CAD build for the part. Positions are in the model's coordinates, mm. A direction names the side the tool comes from. Round coordinates to 2 decimals unless told otherwise and drop trailing zeros. Write each loop counter-clockwise with the first axis right and the second up, starting at its lowest first coordinate (ties: lowest second). Pieces come first, ordered by that corner, then holes. Notation, with made-up numbers: (16, 12.5) - (53, 12.5) arc R19 ccw to (53, 22.5) - close; hole circle Ø1 at (46, 56.5). An arc over 180 degrees is marked (long way). Answer in a Markdown table with one row per item.
```python
from build123d import *

# Parameters (mm, degrees)
SKETCH1_W           = 42.291
SKETCH1_H           = 33.02
BOSS_EXTRUDE1_DEPTH = 42.418
FILLET1_R           = 2.54
SKETCH2_R           = 2.5273
BOSS_EXTRUDE2_DEPTH = 23.9649
CUT_EXTRUDE2_DEPTH  = 18.288
CUT_EXTRUDE3_REACH  = 58.985


with BuildPart() as part:
    # Sketch1 → Boss-Extrude1 (new body)
    with BuildSketch(Plane.XY):
        Rectangle(SKETCH1_W, SKETCH1_H)
    extrude(amount=BOSS_EXTRUDE1_DEPTH)

    # Fillet1
    fillet1_edges = [part.edges().sort_by_distance(p)[0] for p in [
        (21.1455, 0, 42.418),
        (0, 16.51, 42.418),
        (-21.1455, 0, 42.418),
        (0, 16.51, 0),
        (21.1455, 0, 0),
        (0, -16.51, 0),
        (-21.1455, 0, 0),
        (0, -16.51, 42.418),
        (-21.1455, 16.51, 21.209),
        (21.1455, 16.51, 21.209),
        (21.1455, -16.51, 21.209),
        (-21.1455, -16.51, 21.209),
    ]]
    fillet(fillet1_edges, radius=FILLET1_R)

    # Sketch2 → Boss-Extrude2 (add)
    with BuildSketch(Plane(origin=(0, 16.51, 0), x_dir=(1, 0, 0), z_dir=(0, 1, 0))):
        with Locations((0, -21.209)):
            Circle(SKETCH2_R)
    extrude(amount=BOSS_EXTRUDE2_DEPTH)

    # Sketch4 → Cut-Extrude2 (cut)
    with BuildSketch(Plane(origin=(0, 40.4749, 0), x_dir=(1, 0, 0), z_dir=(0, 1, 0))):
        with BuildLine():
            Line((-1.778, -23.005096125), (-1.778, -19.412903875))
            ThreePointArc((-1.778, -19.412903875), (-2.5273, -21.209), (-1.778, -23.005096125))
        make_face()
    extrude(amount=-CUT_EXTRUDE2_DEPTH, mode=Mode.SUBTRACT)

    # Sketch5 → Cut-Extrude3 (cut, up to next)
    with BuildSketch(Plane.XZ.offset(16.51), mode=Mode.PRIVATE) as cut_extrude3_sk1:
        Polygon((-21.1455, 42.418), (-21.1455, 38.107477062), (-16.834977062, 42.418), align=None)
    cut_extrude3_tool1 = extrude(cut_extrude3_sk1.sketch, amount=-CUT_EXTRUDE3_REACH, mode=Mode.PRIVATE) & part.part
    add(cut_extrude3_tool1.solids().sort_by_distance((-19.708659, -16.51, 40.981159))[0], mode=Mode.SUBTRACT)
    # Sketch5 → Cut-Extrude3 (cut, up to next)
    with BuildSketch(Plane.XZ.offset(16.51), mode=Mode.PRIVATE) as cut_extrude3_sk2:
        Polygon((16.961977062, 42.418), (21.2725, 38.107477062), (21.2725, 42.418), align=None)
    cut_extrude3_tool2 = extrude(cut_extrude3_sk2.sketch, amount=-CUT_EXTRUDE3_REACH, mode=Mode.PRIVATE) & part.part
    add(cut_extrude3_tool2.solids().sort_by_distance((19.835659, -16.51, 40.981159))[0], mode=Mode.SUBTRACT)
    # Sketch5 → Cut-Extrude3 (cut, up to next)
    with BuildSketch(Plane.XZ.offset(16.51), mode=Mode.PRIVATE) as cut_extrude3_sk3:
        Polygon((-21.1455, 0), (-16.834977062, 0), (-21.1455, 4.310522938), align=None)
    cut_extrude3_tool3 = extrude(cut_extrude3_sk3.sketch, amount=-CUT_EXTRUDE3_REACH, mode=Mode.PRIVATE) & part.part
    add(cut_extrude3_tool3.solids().sort_by_distance((-19.708659, -16.51, 1.436841))[0], mode=Mode.SUBTRACT)
    # Sketch5 → Cut-Extrude3 (cut, up to next)
    with BuildSketch(Plane.XZ.offset(16.51), mode=Mode.PRIVATE) as cut_extrude3_sk4:
        Polygon((21.2725, 0), (21.2725, 4.310522938), (16.961977062, 0), align=None)
    cut_extrude3_tool4 = extrude(cut_extrude3_sk4.sketch, amount=-CUT_EXTRUDE3_REACH, mode=Mode.PRIVATE) & part.part
    add(cut_extrude3_tool4.solids().sort_by_distance((19.835659, -16.51, 1.436841))[0], mode=Mode.SUBTRACT)


solid = part.part
```
Q1. Saw through at C-C on x = 0. List the corners of the cut face in (y, z).
Computed:
| item | result |
|---|---|
| outline | (-16.51, 2.54) arc R2.54 ccw to (-13.97, 0) - (13.97, 0) arc R2.54 ccw to (16.51, 2.54) - (16.51, 18.68) - (40.47, 18.68) - (40.47, 23.74) - (16.51, 23.74) - (16.51, 39.88) arc R2.54 ccw to (13.97, 42.42) - (-13.97, 42.42) arc R2.54 ccw to (-16.51, 39.88) - close |
Q2. Saw through at B-B on y = -10.5. List the corners of the cut face in (x, z), then the cut area to 3 significant figures.
Computed:
| item | result |
|---|---|
| outline | (-21.15, 4.31) - (-16.83, 0) - (16.96, 0) - (21.15, 4.18) - (21.15, 38.23) - (16.96, 42.42) - (-16.83, 42.42) - (-21.15, 38.11) - close |
| area | 1,760 mm2 |
Q3. Drill centre lines: line 1 (Y direction, x = 15, z = 40.5); line 2 (Y direction, x = 4.5, z = 29.5); line 3 (X direction, y = 4.5, z = 39). Where is each one in solid material? Low to high.
Computed:
| item | result |
|---|---|
| line 1 | y = -16.43 to 16.43 |
| line 2 | y = -16.51 to 16.51 |
| line 3 | x = -20.25 to 20.38 |
Q4. Flat gauge pins, fed straight in: pin 1 (10 mm diameter, centred on x = -16, y = 20.5, fed in from -Z); pin 2 (1.1 mm diameter, centred on y = 31.5, z = 21, fed in from -X); pin 3 (10 mm diameter, centred on x = -15.5, z = 16.5, fed in from +Y); pin 4 (0.6 mm diameter, centred on x = -2, z = 20.5, fed in from +Y). Where does each tip first touch, or does it go through?
Computed:
| item | result |
|---|---|
| pin 1 | stops at z = 0.51 |
| pin 2 | stops at x = -1.78 |
| pin 3 | stops at y = 16.51 |
| pin 4 | stops at y = 40.47 |
Q5. Pull direction X, two halves, no side cores. Call faces 1 (the cylindrical face through (20.38, -15.79, 21.47)), 2 (the flat face through (-19.02, -0.23, 40.233)), 3 (the cylindrical face through (0.26, 15.79, 41.65)): released by +X, released by -X, zero draft, split by the parting line, or undercut.
Computed:
| item | result |
|---|---|
| face 1 | released by +X |
| face 2 | released by -X |
| face 3 | zero draft |
Q6. Saw through at A-A on x = -12. List the corners of the cut face in (y, z), then the cut area to 3 significant figures.
Computed:
| item | result |
|---|---|
| outline | (-16.51, 2.54) arc R2.54 ccw to (-13.97, 0) - (13.97, 0) arc R2.54 ccw to (16.51, 2.54) - (16.51, 39.88) arc R2.54 ccw to (13.97, 42.42) - (-13.97, 42.42) arc R2.54 ccw to (-16.51, 39.88) - close |
| area | 1,400 mm2 |
Q7. 3-axis set-ups, long thin cutter, end or side, ignore diameter. For faces 4 (the flat face through (-1.778, 31, 21)), 5 (the cylindrical face through (2.41, 28.32, 20.45)), 6 (the flat face through (-21.146, 0, 21)): which of +Z, -Z, +X, -X, +Y, -Y reach the whole face in a straight line?
Computed:
| item | result |
|---|---|
| face 4 | +Z, -Z, -X, +Y |
| face 5 | +Y |
| face 6 | +Z, -Z, -X, +Y, -Y |
Q8. Saw through at D-D on y = 31. List the corners of the cut face in (x, z), then the cut area to 3 significant figures.
Computed:
| item | result |
|---|---|
| outline | (-1.78, 19.41) arc R2.53 ccw (long way) to (-1.78, 23.01) - close |
| area | 18.2 mm2 |
